from build123d import *

# Parameters (mm, degrees)
SKETCH3_R           = 17.5
SKETCH3_R_2         = 15.5
BOSS_EXTRUDE1_DEPTH = 150
BOSS_EXTRUDE2_DEPTH = 20
BOSS_EXTRUDE3_DEPTH = 20
SKETCH6_W           = 5
SKETCH6_H           = 5
BOSS_EXTRUDE4_DEPTH = 6
SKETCH7_R           = 1.5
CUT_EXTRUDE2_DEPTH  = 50
SKETCH9_W           = 6
SKETCH9_H           = 10
CUT_EXTRUDE3_DEPTH  = 2
FILLET3_R           = 3.2


with BuildPart() as part:
    # Sketch3 → Boss-Extrude1 (new body)
    with BuildSketch(Plane(origin=(0, 0, 0), x_dir=(1, 0, 0), z_dir=(0, 1, 0))):
        with Locations(Location((0, 0, 0), (0, 0, 270))):
            Circle(SKETCH3_R)
        with Locations(Location((0, 0, 0), (0, 0, 270))):
            Circle(SKETCH3_R_2, mode=Mode.SUBTRACT)
    extrude(amount=BOSS_EXTRUDE1_DEPTH)

    # Sketch4 → Boss-Extrude2 (add)
    with BuildSketch(Plane(origin=(0, 150, 0), x_dir=(1, 0, 0), z_dir=(0, 1, 0))):
        with BuildLine():
            ThreePointArc((17.5, 0), (12.609164887, 12.135030319), (0.670404475, 17.487154081))
            Line((0.670404475, 17.487154081), (0.670404475, 16.661380915))
            Line((0.670404475, 16.661380915), (0.999793375, 16.661380915))
            Line((0.999793375, 16.661380915), (0.999793375, 16.95829018))
            Line((0.999793375, 16.95829018), (1.342992881, 16.95829018))
            Line((1.342992881, 16.95829018), (1.340586782, 15.830625123))
            Line((1.340586782, 15.830625123), (0.65523527, 15.830625123))
            Line((0.65523527, 15.830625123), (0.65523527, 15.486144347))
            ThreePointArc((0.65523527, 15.486144347), (11.189417918, 10.725993038), (15.5, 0))
            Line((15.5, 0), (17.5, 0))
        make_face()
        with BuildLine():
            ThreePointArc((0.670404475, -17.487154081), (12.609164887, -12.135030319), (17.5, 0))
            Line((17.5, 0), (15.5, 0))
            ThreePointArc((15.5, 0), (11.189417918, -10.725993038), (0.65523527, -15.486144347))
            Line((0.65523527, -15.486144347), (0.65523527, -15.830625123))
            Line((0.65523527, -15.830625123), (1.340586782, -15.830625123))
            Line((1.340586782, -15.830625123), (1.342992881, -16.95829018))
            Line((1.342992881, -16.95829018), (0.999793375, -16.95829018))
            Line((0.999793375, -16.95829018), (0.999793375, -16.661380915))
            Line((0.999793375, -16.661380915), (0.670404475, -16.661380915))
            Line((0.670404475, -16.661380915), (0.670404475, -17.487154081))
        make_face()
    extrude(amount=BOSS_EXTRUDE2_DEPTH)

    # Sketch5 → Boss-Extrude3 (add)
    with BuildSketch(Plane(origin=(0, 170, 0), x_dir=(1, 0, 0), z_dir=(0, 1, 0))):
        with BuildLine():
            Line((0.65523527, 15.830625123), (0.65523527, 15.486144347))
            ThreePointArc((0.65523527, 15.486144347), (15.5, 0), (0.65523527, -15.486144347))
            Line((0.65523527, -15.486144347), (0.65523527, -15.830625123))
            Line((0.65523527, -15.830625123), (1.340586782, -15.830625123))
            Line((1.340586782, -15.830625123), (1.342992881, -16.95829018))
            Line((1.342992881, -16.95829018), (0.999793375, -16.95829018))
            Line((0.999793375, -16.95829018), (0.999793375, -16.661380915))
            Line((0.999793375, -16.661380915), (0.670404475, -16.661380915))
            Line((0.670404475, -16.661380915), (0.670404475, -17.487154081))
            ThreePointArc((0.670404475, -17.487154081), (17.5, 0), (0.670404475, 17.487154081))
            Line((0.670404475, 17.487154081), (0.670404475, 16.661380915))
            Line((0.670404475, 16.661380915), (0.999793375, 16.661380915))
            Line((0.999793375, 16.661380915), (0.999793375, 16.95829018))
            Line((0.999793375, 16.95829018), (1.342992881, 16.95829018))
            Line((1.342992881, 16.95829018), (1.340586782, 15.830625123))
            Line((1.340586782, 15.830625123), (0.65523527, 15.830625123))
        make_face()
        with BuildLine():
            ThreePointArc((11.842719282, -10), (15.5, 0), (11.842719282, 10))
            Line((11.842719282, 10), (11.842719282, -10))
        make_face()
    extrude(amount=BOSS_EXTRUDE3_DEPTH)

    # Sketch6 → Boss-Extrude4 (add)
    with BuildSketch(Plane.ZY.offset(-11.842719282)):
        with Locations((-6.2, 177.5)):
            Rectangle(SKETCH6_W, SKETCH6_H)
        with Locations((6.2, 177.5)):
            Rectangle(SKETCH6_W, SKETCH6_H)
    extrude(amount=BOSS_EXTRUDE4_DEPTH)

    # Sketch7 → Cut-Extrude2 (cut)
    with BuildSketch(Plane(origin=(0, 0, -8.7), x_dir=(-1, 0, 0), z_dir=(0, 0, -1))):
        with Locations((-8.842719282, 177.5)):
            Circle(SKETCH7_R)
    extrude(amount=-CUT_EXTRUDE2_DEPTH, mode=Mode.SUBTRACT)

    # Sketch9 → Cut-Extrude3 (cut)
    with BuildSketch(Plane.ZY.offset(-11.842719282)):
        with Locations((0, 177.5)):
            Rectangle(SKETCH9_W, SKETCH9_H)
    extrude(amount=-CUT_EXTRUDE3_DEPTH, mode=Mode.SUBTRACT)

    # Fillet3
    # the kernel refuses this fillet: 3.2 mm, written as the material it adds along each edge
    with BuildSketch(Plane(origin=(13.842719282, 172.5, -3), x_dir=(-1, 0, 0), z_dir=(0, 1, 0)), Plane(origin=(13.842719282, 189.916198487, 3), x_dir=(-1, 0, 0), z_dir=(0, -1, 0))) as fillet3_piece_1:
        with BuildLine():
            CenterArc((3.2, 2.966479395), FILLET3_R, 180, 67.975687163)
            Line((0, 2.966479395), (-0.064, 2.966479395))
            Line((-0.064, 2.966479395), (-0.064, 0))
            Line((-0.064, 0), (0, -0.064))
            ThreePointArc((0, -0.064), (1, -0.064), (1.976, -0.059329588))
            Line((1.976, -0.059329588), (2, 0))
        make_face()
    extrude(amount=17.416198487)
    with BuildSketch(Plane(origin=(13.842719282, 172.5, 10.416198487), x_dir=(-1, 0, 0), z_dir=(0, 0, -1)), Plane(origin=(13.842719282, 182.5, -10.416198487), x_dir=(-1, 0, 0), z_dir=(0, 0, 1))) as fillet3_piece_2:
        with BuildLine():
            CenterArc((3.2, 2.966479395), FILLET3_R, 180, 67.975687163)
            Line((0, 2.966479395), (-0.064, 2.966479395))
            Line((-0.064, 2.966479395), (-0.064, 0))
            Line((-0.064, 0), (0, -0.064))
            ThreePointArc((0, -0.064), (1, -0.064), (1.976, -0.059329588))
            Line((1.976, -0.059329588), (2, 0))
        make_face()
    extrude(amount=20.832396974)


solid = part.part
Source: CAD feature listing. Evaluate the final solid. Frame: model axes, mm. A direction names the side the tool comes from. Give positions to 0.01 mm unless a question says otherwise; leave off trailing zeros. Write each loop counter-clockwise with the first axis right and the second up, starting at its lowest first coordinate (ties: lowest second). Pieces come first, ordered by that corner, then holes. Notation, with made-up numbers: M 51,21 L 88,21 A19 cw 88,28 Z; hole C -23,15 d8. An arc over 180 degrees is marked long. Return JSON: item names as keys, results as strings. Group by question number.
1) Cut plane A-A, the plane z = -5.5. Output: boundary loops of the cut face in (x, y), then the cut area to 3 significant figures.
2) Cut plane D-D, the plane z = -13.5. Output: boundary loops of the cut face in (x, y).
3) First-contact query: pin 1 Ø2 at (x, y) = (-0.5, 137.5) entering from -Z; pin 2 Ø2.5 at (x, y) = (8.84, 177.5) entering from -Z; pin 3 Ø1.5 at (x, y) = (9, 178.5) entering from +Z; pin 4 Ø3 at (y, z) = (134.5, 13.5) entering from +X. Flat tips, straight axial feed; report the tip coordinate or a pass-through.
4) Cut plane C-C, the plane y = 103. Output: boundary loops of the cut face in (x, z).
5) Set-up query: faces 1 (the face through (9, 180, 6)), 2 (the face through (12, 190, -1)), 3 (the face through (9, 175, 6)), 4 (the face through (13.055, 177.57, 2.136)), 5 (the face through (5.843, 178, -6)). Return all of +Z, -Z, +X, -X, +Y, -Y with unobstructed straight access to the full face (end or side cutting, diameter ignored); none if empty.
6) Cut plane B-B, the plane x = -6.5. Output: boundary loops of the cut face in (y, z).
7) Draft query along X for faces 6 (the face through (10.033, 176.587, 13.684)), 7 (the face through (8.9, 175.8, -3.7)), 8 (the face through (13.055, 177.43, -2.136)), 9 (the face through (8.036, 178.765, -6.235)). Return one class per face: released by +X, released by -X, zero draft, split by the parting line, or undercut.
8) Ray query, L1, parallel to Z at x = -0.5, y = 94; L2, parallel to X at y = 91.5, z = -1; L3, parallel to Y at x = 9, z = 6. Return the intervals inside material, ascending.
Data:
{
 "1": {"outline": "M -16.61,0 L -14.49,0 L -14.49,150 L -16.61,150 Z; M 5.84,175 L 11.84,175 L 11.84,170 L 14.49,170 L 14.49,0 L 16.61,0 L 16.61,190 L 11.84,190 L 11.84,180 L 5.84,180 Z; hole C 8.84,177.5 d3", "area": "797 mm²"},
 "2": {"outline": "M -11.14,0 L -7.62,0 L -7.62,150 L -11.14,150 Z; M 7.62,0 L 11.14,0 L 11.14,190 L 7.62,190 Z"},
 "3": {"pin 1": "stops at z = -17.5", "pin 2": "stops at z = -15.77", "pin 3": "stops at z = 15.36", "pin 4": "stops at x = 12.74"},
 "4": {"outline": "C 0,0 d35; hole C 0,0 d31"},
 "5": {"face 1": "-X, +Y", "face 2": "+Z, -Z, +X, -X, +Y", "face 3": "-X, -Y", "face 4": "-X", "face 5": "-X, +Y, -Y"},
 "6": {"outline": "M 0,-16.25 L 150,-16.25 L 150,-14.07 L 0,-14.07 Z; M 0,14.07 L 150,14.07 L 150,16.25 L 0,16.25 Z"},
 "7": {"face 6": "undercut", "face 7": "zero draft", "face 8": "released by -X", "face 9": "undercut"},
 "8": {"L1": "z = -17.49 to -15.49, 15.49 to 17.49", "L2": "x = -17.47 to -15.47, 15.47 to 17.47", "L3": "y = 175 to 176.01, 178.99 to 180"}
}
